The model under review builds one solid part; all positions refer to its coordinate system, in mm. Face numbers are marked on the shaded views. A direction names the side the tool comes from. Round coordinates to 2 decimals unless told otherwise and drop trailing zeros. Write each loop counter-clockwise with the first axis right and the second up, starting at its lowest first coordinate (ties: lowest second). Pieces come first, ordered by that corner, then holes.
Item 1: Add section C-C (z = 19). Give the boundary of the cut face in (x, y).
Item 2: Draft analysis for pull direction Y (two halves, no side actions). For the marked faces 1, 2 and 3, state which applies: +Y half, -Y half, draft (parallel to the pull), parting line (faces both ways), or undercut.
Item 3: Clearance check with flat-ended pins moving along their axes: pin 1 Ø8 at (x, z) = (-30.5, 29.5) entering from +Y; pin 2 Ø10 at (x, y) = (-36, 30) entering from +Z; pin 3 Ø10 at (y, z) = (-17, 19.5) entering from +X; pin 4 Ø8 at (x, y) = (31.5, -11.5) entering from +Z. State where each tip first meets the part, or that it passes through.
Item 4: Add section D-D (z = 42.5). Give the boundary of the cut face in (x, y), plus the area to 3 significant figures.
Item 5: Machinability: for the marked faces 4 and 5, which of the approach directions +Z, -Z, +X, -X, +Y, -Y give a long, thin tool a straight path to every point of the face, cutting with its end or side? Answer none if there is none.
Item 6: To check wall thickness, follow L1, parallel to Y at x = 0, z = 30; L2, parallel to Y at x = -9.5, z = 31; L3, parallel to X at y = 1, z = 34.5. State the ranges of each line that lie inside material, in increasing order.
Item 7: Add section A-A (x = 0). Give the boundary of the cut face in (y, z), plus the area to 3 significant figures.
Solid Edge part; units mm, degrees
sketch "Sketch1" plane through (0, 0, 0) normal (0, -1, 0) x (1, 0, 0)
  arc A0 (25, 51.8641) -> (30, 46.8641) centre (30, 51.8641) ccw
  line L0 (30, 46.8641) -> (40, 46.8641)
  arc A1 (40, 46.8641) -> (40, 36.8641) centre (40, 41.8641) cw
  line L1 (40, 36.8641) -> (25, 36.8641)
  line L2 (25, 36.8641) -> (25, 11.8641)
  line L3 (25, 11.8641) -> (15, 11.8641)
  line L4 (15, 11.8641) -> (15, 56.8641)
  line L5 (15, 56.8641) -> (25, 56.8641)
  line L6 (25, 56.8641) -> (25, 51.8641)
revolve "RevolvedProtrusion1" add sketch "Sketch1" angle 360 about axis through (0, 0, 0) along (0, 0, 1)
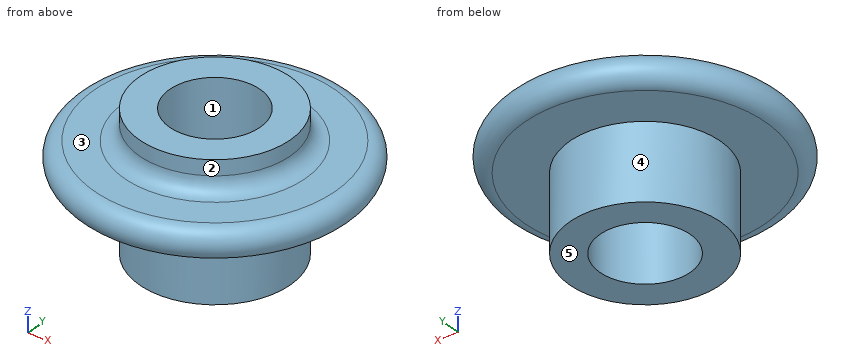
Numbers:
1. outline: circle Ø50 at (0, 0); hole circle Ø30 at (0, 0)
2. face 1: undercut
2. face 2: parting line
2. face 3: draft
3. pin 1: passes through
3. pin 2: stops at z = 46.5
3. pin 3: stops at x = 21.93
3. pin 4: stops at z = 46.89
4. outline: circle Ø89.92 at (0, 0); hole circle Ø30 at (0, 0)
4. area: 5,640 mm2
5. face 4: -Z
5. face 5: -Z, +X, -X, +Y, -Y
6. L1: y = -25 to -15, 15 to 25
6. L2: y = -23.12 to -11.61, 11.61 to 23.12
6. L3: x = -24.98 to -14.97, 14.97 to 24.98
7. outline: (-40, 36.86) - (-25, 36.86) - (-25, 11.86) - (-15, 11.86) - (-15, 56.86) - (-25, 56.86) - (-25, 51.86) arc R5 cw to (-30, 46.86) - (-40, 46.86) arc R5 ccw to start; (15, 11.86) - (25, 11.86) - (25, 36.86) - (40, 36.86) arc R5 ccw to (40, 46.86) - (30, 46.86) arc R5 cw to (25, 51.86) - (25, 56.86) - (15, 56.86) - close
7. area: 1,290 mm2
